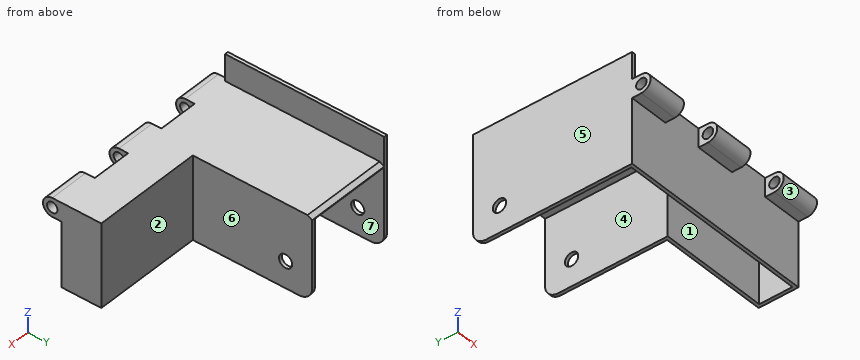
from build123d import *

# Parameters (mm, degrees)
F0_W      = 3.175
F0_H      = 76.2
F0_H_2    = 3.175
F0_W_2    = 79.375
F1_DEPTH  = 152.4
F2_W      = 3.175
F2_H      = 76.2
F2_H_2    = 3.175
F2_W_2    = 31.75
F3_DEPTH  = 76.2
F4_W      = 3.175
F4_H      = 76.2
F5_DEPTH  = 79.375
F6_W      = 3.175
F6_H      = 76.2
F7_DEPTH  = 31.75
F8_R      = 5.0419
F9_DEPTH  = 161.925
F11_DEPTH = 17.781
F12_DEPTH = 61.596
F13_W     = 3.175
F13_H     = 152.4
F14_DEPTH = 25.4
F15_DEPTH = 25.4
F16_R     = 6.35
F17_DEPTH = 85.726
F18_R     = 12.7
F19_SIZE2 = 4.3994090512
F19_SIZE  = 2.54
F20_DEPTH = 38.1
F21_W     = 3.175
F21_H     = 76.2
F22_DEPTH = 31.75
F23_DEPTH = 28.575
F24_DEPTH = 9.525


with BuildPart() as f1:
    # F0 (on Front) → F1 (new body)
    with BuildSketch(Plane.XZ):
        with Locations((1.5875, 38.1)):
            Rectangle(F0_W, F0_H)
        with Locations((1.5875, 77.7875)):
            Rectangle(F0_W, F0_H_2)
        with Locations((42.8625, 77.7875)):
            Rectangle(F0_W_2, F0_H_2)
        with Locations((84.1375, 77.7875)):
            Rectangle(F0_W, F0_H_2)
        with Locations((84.1375, 38.1)):
            Rectangle(F0_W, F0_H)
    extrude(amount=F1_DEPTH)

    # F2 (on face) → F3 (join)
    with BuildSketch(Plane.YZ.offset(85.725)):
        with Locations((-150.8125, 38.1)):
            Rectangle(F2_W, F2_H)
        with Locations((-150.8125, 77.7875)):
            Rectangle(F2_W, F2_H_2)
        with Locations((-133.35, 77.7875)):
            Rectangle(F2_W_2, F2_H_2)
        with Locations((-115.8875, 38.1)):
            Rectangle(F2_W, F2_H)
        with Locations((-115.8875, 77.7875)):
            Rectangle(F2_W, F2_H_2)
    extrude(amount=F3_DEPTH)

    # F4 (on face) → F5 (join, through all)
    with BuildSketch(Plane.YZ.offset(3.175)):
        with Locations((-150.8125, 38.1)):
            Rectangle(F4_W, F4_H)
    extrude(amount=F5_DEPTH)

    # F6 (on face) → F7 (join, through all)
    with BuildSketch(Plane.XZ.offset(117.475)):
        with Locations((160.3375, 38.1)):
            Rectangle(F6_W, F6_H)
    extrude(amount=F7_DEPTH)

    # F8 (on face) → F9 (join, through all)
    with BuildSketch(Plane.YZ.offset(161.925)):
        with BuildLine():
            Line((-152.4, 79.375), (-161.29, 79.375))
            ThreePointArc((-161.29, 79.375), (-170.18, 70.485), (-161.29, 61.595))
            Line((-161.29, 61.595), (-152.4, 61.595))
            Line((-152.4, 61.595), (-152.4, 79.375))
        make_face()
        with Locations((-161.29, 70.485)):
            Circle(F8_R, mode=Mode.SUBTRACT)
    extrude(amount=-F9_DEPTH)

    # F10 (on face) → F11 (cut, through all)
    with BuildSketch(Plane(origin=(0, 0, 61.595), x_dir=(1, 0, 0), z_dir=(0, 0, -1))):
        Polygon((114.3, 152.4), (152.4, 152.4), (152.4, 171.5404093266), (152.4, 189.2811655998), (114.3, 189.2811655998), (114.3, 183.5609525442), align=None)
        Polygon((152.4, 171.5404093266), (152.4, 152.4), (152.4, 103.7641689181), (174.3682473898, 103.7641689181), (174.3682473898, 171.5404093266), align=None)
        Polygon((38.1, 152.4), (76.2, 152.4), (76.2, 183.5609525442), (76.2, 185.6450736523), (38.1, 185.6450736523), (38.1, 184.6726387739), align=None)
    extrude(amount=-F11_DEPTH, mode=Mode.SUBTRACT)

    # F12 (cut, through all): a face of the model
    f12_faces = [f1.faces().sort_by_distance(p)[0] for p in [
        (159.146875, -133.35, 61.595),
    ]]
    extrude(f12_faces, amount=-F12_DEPTH, mode=Mode.SUBTRACT)

    # F13 (on face) → F14 (join)
    with BuildSketch(Plane.XY.offset(79.375)):
        with Locations((1.5875, -76.2)):
            Rectangle(F13_W, F13_H)
    extrude(amount=F14_DEPTH)

    # F15 (cut): a face of the model
    f15_faces = [f1.faces().sort_by_distance(p)[0] for p in [
        (85.725, -133.35, 38.1),
    ]]
    extrude(f15_faces, amount=-F15_DEPTH, mode=Mode.SUBTRACT)

    # F16 (on face) → F17 (cut, through all)
    with BuildSketch(Plane.YZ.offset(85.725)):
        with Locations((-25.4, 25.4)):
            Circle(F16_R)
    extrude(amount=-F17_DEPTH, mode=Mode.SUBTRACT)

    # F18
    f18_edges = [f1.edges().sort_by_distance(p)[0] for p in [
        (84.1375, 0, 0),
        (1.5875, 0, 0),
    ]]
    fillet(f18_edges, radius=F18_R)

    # F19
    f19_edges = [f1.edges().sort_by_distance(p)[0] for p in [
        (44.45, 0, 79.375),
    ]]
    f19_side = f1.faces().sort_by_distance((1.916963, 0, 44.45))[0]
    chamfer(f19_edges, length=F19_SIZE, length2=F19_SIZE2, reference=f19_side)

    # F20 (add): a face of the model
    f20_faces = [f1.faces().sort_by_distance(p)[0] for p in [
        (152.4, -115.1804544636, 39.6875),
    ]]
    extrude(f20_faces, amount=F20_DEPTH)

    # F21 (on face) → F22 (join, through all)
    with BuildSketch(Plane.XZ.offset(117.475)):
        with Locations((188.9125, 38.1)):
            Rectangle(F21_W, F21_H)
    extrude(amount=F22_DEPTH)

    # F8 (on face) → F23 (join, through all)
    with BuildSketch(Plane.YZ.offset(161.925)):
        with BuildLine():
            Line((-152.4, 79.375), (-161.29, 79.375))
            ThreePointArc((-161.29, 79.375), (-170.18, 70.485), (-161.29, 61.595))
            Line((-161.29, 61.595), (-152.4, 61.595))
            Line((-152.4, 61.595), (-152.4, 79.375))
        make_face()
        with Locations((-161.29, 70.485)):
            Circle(F8_R, mode=Mode.SUBTRACT)
    extrude(amount=F23_DEPTH)

    # F24 (add): a face of the model
    f24_faces = [f1.faces().sort_by_distance(p)[0] for p in [
        (161.925, -156.845, 61.8464471714),
    ]]
    extrude(f24_faces, amount=F24_DEPTH)


solid = f1.part
Design review of the part built by this model. Coordinates are the model's own, in mm. Face numbers are marked on the shaded views. A direction names the side the tool comes from. Give positions to 0.01 mm unless a question says otherwise; leave off trailing zeros. Write each loop counter-clockwise with the first axis right and the second up, starting at its lowest first coordinate (ties: lowest second). Pieces come first, ordered by that corner, then holes. Notation, with made-up numbers: M 4,33 L 10,33 A16 ccw 10,42 Z; hole C 86,-15.75 d1. An arc over 180 degrees is marked long. Answer as a JSON object with one key per item and string values. Group by question number.
1) For line 1 along Y through (x, z) = (156.5, 44.5) (3 decimals); line 2 along X through (y, z) = (-54.5, 37.5) (3 decimals); line 3 along Y through (x, z) = (83, 25) (3 decimals), list the stretches that pass through material, from the lowest coordinate up.
2) Mouldability with a two-part tool opening along X and no side actions: class the marked faces 4, 5, 6 and 7 as released by +X, released by -X, zero draft, split by the parting line, or undercut.
3) We need section C-C (y = -60.5). Give the boundary of the cut face in (x, z) (3 decimals), and give its area (3 significant figures).
4) We need section A-A (y = -25.4). Give the boundary of the cut face in (x, z) (3 decimals), and give its area (3 significant figures).
5) We need section D-D (y = -134). Give the boundary of the cut face in (x, z) (3 decimals), and give its area (3 significant figures).
6) Clearance check with flat-ended pins moving along their axes: pin 1 Ø5 at (x, z) = (86.5, 19.5) entering from -Y; pin 2 Ø22.5 at (y, z) = (-97.5, 94) entering from +X (3 decimals); pin 3 Ø8 at (x, y) = (45, -24) entering from -Z. State where each tip first meets the part, or that it passes through.
7) We need section B-B (z = 25.4). Give the boundary of the cut face in (x, y) (3 decimals), and give its area (3 significant figures).
8) Tool access review of the marked faces 1, 2 and 3: name each direction out of +Z, -Z, +X, -X, +Y, -Y from which nothing blocks a thin tool from reaching the whole face with its end or side.
Answer key:
{
 "1": {"line 1": "y = -152.4 to -149.225, -117.475 to -114.3", "line 2": "x = 0 to 3.175, 82.55 to 85.725", "line 3": "y = -152.4 to -149.225, -117.475 to -31.737, -19.063 to 0"},
 "2": {"face 4": "undercut", "face 5": "released by -X", "face 6": "released by +X", "face 7": "undercut"},
 "3": {"outline": "M 0,0 L 3.175,0 L 3.175,76.2 L 82.55,76.2 L 82.55,0 L 85.725,0 L 85.725,79.375 L 3.175,79.375 L 3.175,104.775 L 0,104.775 Z", "area": "837 mm²"},
 "4": {"outline": "M 0,0 L 3.175,0 L 3.175,19.05 L 0,19.05 Z; M 0,31.75 L 3.175,31.75 L 3.175,76.2 L 82.55,76.2 L 82.55,31.75 L 85.725,31.75 L 85.725,79.375 L 3.175,79.375 L 3.175,104.775 L 0,104.775 Z; M 82.55,0 L 85.725,0 L 85.725,19.05 L 82.55,19.05 Z", "area": "756 mm²"},
 "5": {"outline": "M 0,0 L 3.175,0 L 3.175,76.2 L 187.325,76.2 L 187.325,0 L 190.5,0 L 190.5,79.375 L 3.175,79.375 L 3.175,104.775 L 0,104.775 Z", "area": "1,170 mm²"},
 "6": {"pin 1": "stops at y = -152.4", "pin 2": "stops at x = 3.175", "pin 3": "stops at z = 76.2"},
 "7": {"outline": "M 0,-152.4 L 190.5,-152.4 L 190.5,-114.3 L 85.725,-114.3 L 85.725,-31.75 L 82.55,-31.75 L 82.55,-117.475 L 187.325,-117.475 L 187.325,-149.225 L 3.175,-149.225 L 3.175,-31.75 L 0,-31.75 Z; M 0,-19.05 L 3.175,-19.05 L 3.175,0 L 0,0 Z; M 82.55,-19.05 L 85.725,-19.05 L 85.725,0 L 82.55,0 Z", "area": "1,800 mm²"},
 "8": {"face 1": "-Z", "face 2": "+Z, -Z, +X, +Y", "face 3": "+X, -X, -Y"}
}
